Autodesk Inventor part; units mm, degrees
ref_plane "YZ Plane" through (0, 0, 0) normal (1, 0, 0) x (0, 1, 0)
ref_plane "XZ Plane" through (0, 0, 0) normal (0, 1, 0) x (-1, 0, 0)
ref_plane "XY Plane" through (0, 0, 0) normal (0, 0, 1) x (1, 0, 0)
sketch "Sketch1" plane through (0, 0, 0) normal (0, 1, 0) x (-1, 0, 0)
  line L0 (0, -5) -> (-4.3301, -2.5)
  line L1 (-4.3301, -2.5) -> (-4.3301, 2.5)
  line L2 (-4.3301, 2.5) -> (0, 5)
  line L3 (0, 5) -> (4.3301, 2.5)
  line L4 (4.3301, 2.5) -> (4.3301, -2.5)
  line L5 (4.3301, -2.5) -> (0, -5)
  point P0 (0, 0)
  point P1 (0, 0)
  point P2 (0, 0)
  dimension "d1" = 5
extrude "Extrusion1" add sketch "Sketch1" along normal blind 10
sketch "Sketch2" plane through (0, 10, 0) normal (0, 1, 0) x (1, 0, 0)
  circle A0 centre (0, 0) radius 1.5
  dimension "d4" = 3
extrude "Extrusion2" add sketch "Sketch2" along normal blind 6
sketch "Sketch3" plane through (0, 0, 0) normal (0, -1, 0) x (1, 0, 0)
  circle A0 centre (0, 0) radius 1.5
  dimension "d7" = 3
extrude "Extrusion3" add sketch "Sketch3" along normal blind 5
thread "Thread1"
thread "Thread2"
properties part number "spacer" material "Aluminum 6061"
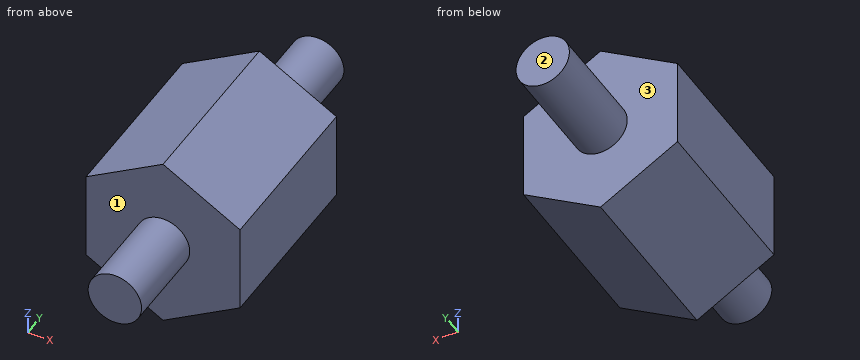
Check sheet for the modelled part. Datum: model origin and axes. Units: mm. Face numbers are marked on the shaded views. A direction names the side the tool comes from. Round coordinates to 2 decimals unless told otherwise and drop trailing zeros. Loops run counter-clockwise (first coordinate to the right, second up) from the corner with the lowest first, then second, coordinate; pieces in that order, holes last.
1. Scan lines: probe 1 along Y at (x, z) = (-1.5, 0.5); probe 2 along Z at (x, y) = (0, -4). Record each from-to range of solid material in increasing order.
2. Sectioned sample at B-B on y = 9.25. Record the boundary of the cut face in (x, z).
3. Gauge pin test, flat end, axial feed: pin 1 Ø1 at (x, z) = (1, -1.5) entering from -Y. Record the tip position at first contact, or that the pin passes through.
4. Sectioned sample at D-D on z = 2. Record the boundary of the cut face in (x, y).
5. Set-up check for the marked faces 1, 2 and 3: record each of +Z, -Z, +X, -X, +Y, -Y from which the full face is reachable in a straight line by a thin tool's end or side.
6. Sectioned sample at A-A on z = 0. Record the boundary of the cut face in (x, y).
7. Sectioned sample at C-C on x = 0.25. Record the boundary of the cut face in (y, z).
Recorded:
1. probe 1: y = 0 to 10
1. probe 2: z = -1.5 to 1.5
2. outline: (-4.33, -2.5) - (0, -5) - (4.33, -2.5) - (4.33, 2.5) - (0, 5) - (-4.33, 2.5) - close
3. pin 1: stops at y = -5
4. outline: (-4.33, 0) - (4.33, 0) - (4.33, 10) - (-4.33, 10) - close
5. face 1: -Y
5. face 2: +Z, -Z, +X, -X, +Y
5. face 3: +Y
6. outline: (-4.33, 0) - (-1.5, 0) - (-1.5, -5) - (1.5, -5) - (1.5, 0) - (4.33, 0) - (4.33, 10) - (1.5, 10) - (1.5, 16) - (-1.5, 16) - (-1.5, 10) - (-4.33, 10) - close
7. outline: (-5, -1.48) - (0, -1.48) - (0, -4.86) - (10, -4.86) - (10, -1.48) - (16, -1.48) - (16, 1.48) - (10, 1.48) - (10, 4.86) - (0, 4.86) - (0, 1.48) - (-5, 1.48) - close
